For this review, use the dimensioned drawing (mm, ordinates from the lowest corner) and the shaded views. Round coordinates to 2 decimals unless told otherwise and drop trailing zeros. Loops run counter-clockwise (first coordinate to the right, second up) from the corner with the lowest first, then second, coordinate; pieces in that order, holes last. Notation, with made-up numbers: (8.5, 51.25) -> (49.5, 51.25) arc R14 cw to (49.5, 67.25) -> close; hole circle Ø5 at (59.25, 78.25). An arc over 180 degrees is marked (long way). Use one line per item in the form item = value. Start each with the question number.
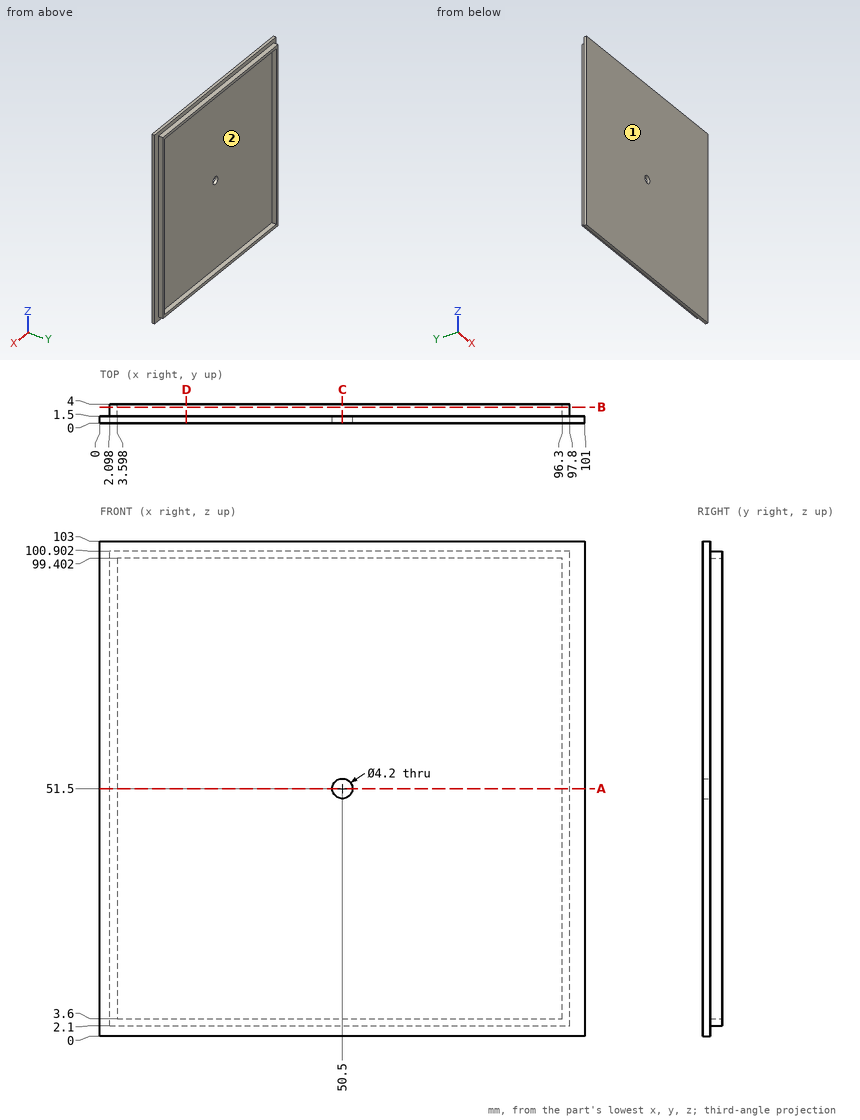
Item 1: For P1, Ø1.2, axis at x = 53.5, y = 2.5, coming from the -Z side; P2, Ø1.2, axis at x = 32.5, y = 2.5, coming from the +Z side; P3, Ø1.2, axis at y = 3, z = 29.5, coming from the -X side, all flat-tipped, find the tip position at first contact; note any pin that passes through.
Item 2: Take a section at C-C on x = 50.5. Give the boundary of the cut face in (y, z), plus the area to 3 significant figures.
Item 3: Take a section at A-A on z = 51.5. Give the boundary of the cut face in (x, y).
Item 4: Take a section at B-B on y = 3.35. Give the boundary of the cut face in (x, z).
Item 5: Draft analysis for pull direction Z (two halves, no side actions). For the marked faces 1 and 2, state which applies: +Z half, -Z half, draft (parallel to the pull), parting line (faces both ways), or undercut.
Item 6: Take a section at D-D on x = 18. Give the boundary of the cut face in (y, z), plus the area to 3 significant figures.
Item 7: Wall thickness on line 1 (Z direction, x = 56, y = 1.75); line 2 (X direction, y = 0.4, z = 51.5); line 3 (X direction, y = 3.8, z = 64.5): over which ranges is each line inside the solid? List them lowest first.
Results:
q1.P1 = 2.1
q1.P2 = 100.9
q1.P3 = 2.1
q2.outline = (0, 0) -> (1.5, 0) -> (1.5, 2.1) -> (4, 2.1) -> (4, 3.6) -> (1.5, 3.6) -> (1.5, 49.4) -> (0, 49.4) -> close; (0, 53.6) -> (1.5, 53.6) -> (1.5, 99.4) -> (4, 99.4) -> (4, 100.9) -> (1.5, 100.9) -> (1.5, 103) -> (0, 103) -> close
q2.area = 156 mm2
q3.outline = (0, 0) -> (48.4, 0) -> (48.4, 1.5) -> (3.6, 1.5) -> (3.6, 4) -> (2.1, 4) -> (2.1, 1.5) -> (0, 1.5) -> close; (52.6, 0) -> (101, 0) -> (101, 1.5) -> (97.8, 1.5) -> (97.8, 4) -> (96.3, 4) -> (96.3, 1.5) -> (52.6, 1.5) -> close
q4.outline = (2.1, 2.1) -> (97.8, 2.1) -> (97.8, 100.9) -> (2.1, 100.9) -> close; hole (3.6, 3.6) -> (96.3, 3.6) -> (96.3, 99.4) -> (3.6, 99.4) -> close
q5.face_1 = draft
q5.face_2 = undercut
q6.outline = (0, 0) -> (1.5, 0) -> (1.5, 2.1) -> (4, 2.1) -> (4, 3.6) -> (1.5, 3.6) -> (1.5, 99.4) -> (4, 99.4) -> (4, 100.9) -> (1.5, 100.9) -> (1.5, 103) -> (0, 103) -> close
q6.area = 162 mm2
q7.line_1 = 2.1 to 3.6, 99.4 to 100.9
q7.line_2 = 0 to 48.4, 52.6 to 101
q7.line_3 = 2.1 to 3.6, 96.3 to 97.8
